```python
from build123d import *

# Parameters (mm, degrees)
SKETCH_1_R          = 12
EXTRUDE_1_DEPTH     = 44
SKETCH_2_R          = 6.5
EXTRUDE_2_DEPTH     = 2
SKETCH_3_R          = 3
EXTRUDE_3_DEPTH     = 15
SKETCH_4_R          = 1.5
CUT_EXTRUDE_1_DEPTH = 5
CUT_EXTRUDE_START   = -11.5
CUT_EXTRUDE_2_DEPTH = 11.5
SKETCH_6_R          = 1.5
CUT_EXTRUDE_3_DEPTH = 48.977426709
FILLET_1_R          = 3


with BuildPart() as part:
    # 草图1 → 凸台-拉伸1 (new body)
    with BuildSketch(Plane.XY):
        Circle(SKETCH_1_R)
    extrude(amount=EXTRUDE_1_DEPTH)

    # 草图2 → 凸台-拉伸2 (add)
    with BuildSketch(Plane(origin=(0, 0, 0), x_dir=(-1, 0, 0), z_dir=(0, 0, -1))):
        Circle(SKETCH_2_R)
    extrude(amount=EXTRUDE_2_DEPTH)

    # 草图3 → 凸台-拉伸3 (add)
    with BuildSketch(Plane(origin=(0, 0, -2), x_dir=(-1, 0, 0), z_dir=(0, 0, -1))):
        Circle(SKETCH_3_R)
    extrude(amount=EXTRUDE_3_DEPTH)

    # 草图4 → 切除-拉伸1 (cut)
    with BuildSketch(Plane(origin=(0, 0, 0), x_dir=(-1, 0, 0), z_dir=(0, 0, -1))):
        with Locations((0, -9)):
            Circle(SKETCH_4_R)
        with Locations((-7.794228634, 4.5)):
            Circle(SKETCH_4_R)
        with Locations((7.794228634, 4.5)):
            Circle(SKETCH_4_R)
    extrude(amount=-CUT_EXTRUDE_1_DEPTH, mode=Mode.SUBTRACT)

    # 草图5 → 切除-拉伸2 (cut)
    with BuildSketch(Plane(origin=(0, 0, -17), x_dir=(-1, 0, 0), z_dir=(0, 0, -1)).offset(CUT_EXTRUDE_START)):
        with BuildLine():
            Line((2.160985852, -2.08089888), (-1.076716839, -2.800121578))
            ThreePointArc((-1.076716839, -2.800121578), (0.650561408, -2.928612275), (2.160985852, -2.08089888))
        make_face()
    extrude(amount=CUT_EXTRUDE_2_DEPTH, mode=Mode.SUBTRACT)

    # 草图6 → 切除-拉伸3 (cut, through all)
    with BuildSketch(Plane(origin=(-0.542134506, -2.440510229, 0), x_dir=(-0.9762040915238366, 0.2168538025770379, 0), z_dir=(-0.2168538025770379, -0.9762040915238366, 0))):
        with Locations(Location((0, 8, 0), (0, 0, 180))):
            Circle(SKETCH_6_R)
    extrude(amount=-CUT_EXTRUDE_3_DEPTH, mode=Mode.SUBTRACT)

    # 圆角1
    fillet_1_edges = [part.edges().sort_by_distance(p)[0] for p in [
        (-12, 0, 44),
    ]]
    fillet(fillet_1_edges, radius=FILLET_1_R)


solid = part.part
```
Check sheet for the modelled part. Datum: model origin and axes. Units: mm. A direction names the side the tool comes from. Coordinates: 2 decimals unless noted, no trailing zeros. Order: outer loops, then holes, each group sorted by start corner. A loop starts at its lowest first (then second) coordinate and runs counter-clockwise, first axis right, second up. Notation, with made-up numbers: M 88,-9 L 111,-9 A17 cw 111,24 Z; hole C 16,86.5 d1. An arc over 180 degrees is marked long. Write each question's results on one line, items separated by ' | '. Start each with the question number.
1. Mould release check, pull along Y, two halves, no side actions. Record for faces 3 (the face through (-11.99, 0.53, 20.21)), 4 (the face through (-0.565, -2.435, -12.447)), 5 (the face through (5, -5, 0)), 6 (the face through (0.325, -10.464, 2.465)): +Y half, -Y half, draft (parallel to the pull), parting line (faces both ways), or undercut.
2. Access from +Z, -Z, +X, -X, +Y, -Y to the whole of each face (thin tool, end or side, straight path). Record for faces 1 (the face through (8, 5, 5)), 2 (the face through (0, 0, 44)).
3. Go/stop test with flat-tipped pins: P1, Ø0.9, axis at x = -7.5, y = 4, coming from the -Z side; P2, Ø3, axis at x = 7.5, z = 10.5, coming from the +Y side; P3, Ø6, axis at x = -4, y = -7.5, coming from the -Z side. Record where each tip stops, or that it passes through.
4. Material ranges on probe 1 along Y at (x, z) = (0, 3.15); probe 2 along Y at (x, z) = (9, 3); probe 3 along Z at (x, y) = (4.75, 7), recorded low to high.
5. Cross-section at A-A on z = 15.5. Record the cut outline in (x, y), and give its area (3 significant figures).
Checks:
1) face 3: parting line | face 4: -Y half | face 5: draft | face 6: undercut
2) face 1: -Z | face 2: +Z, +X, -X, +Y, -Y
3) P1: stops at z = 5 | P2: stops at y = 10.39 | P3: stops at z = -2
4) probe 1: y = -12 to -10.5, -7.5 to 12 | probe 2: y = -7.94 to 3.61, 5.39 to 7.94 | probe 3: z = 0 to 44
5) outline: C 0,0 d24 | area: 452 mm²
